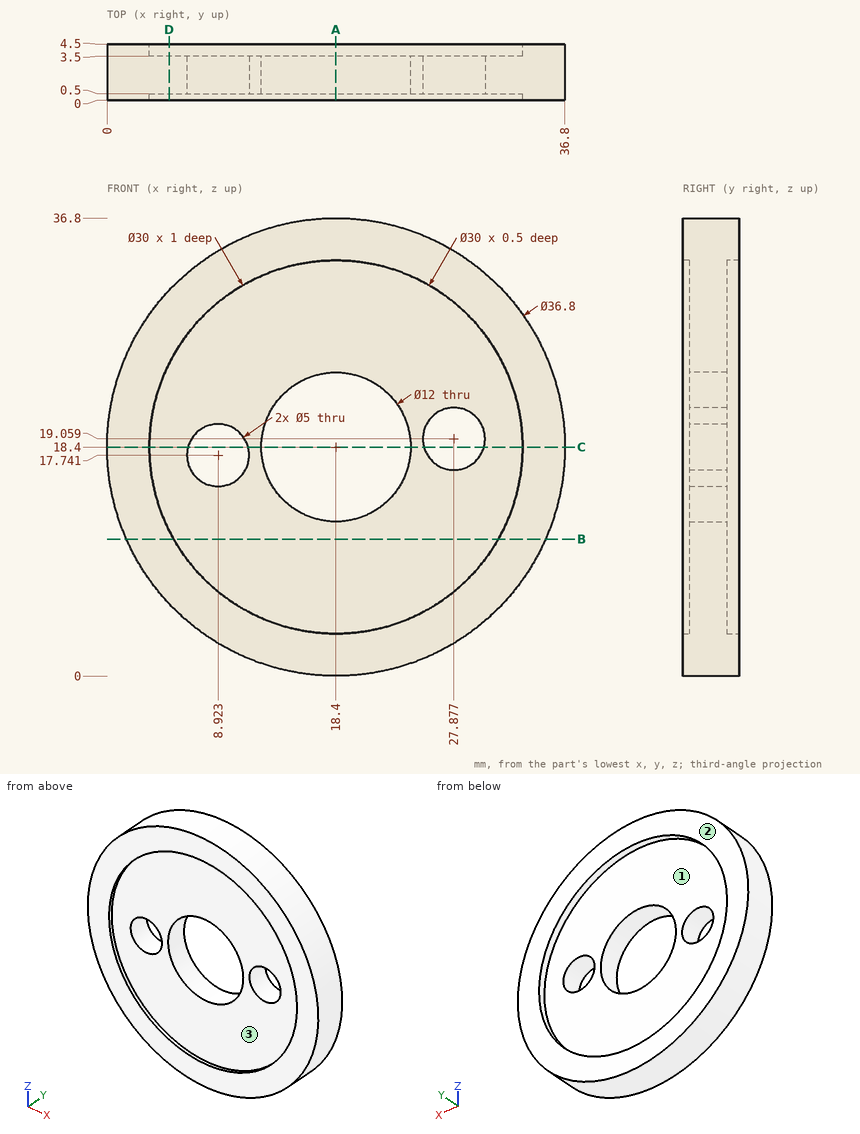
The drawing under review shows one solid part. Ordinate dimensions are in mm from its lowest x, y, z. A direction names the side the tool comes from. Round coordinates to 2 decimals unless told otherwise and drop trailing zeros. Loops run counter-clockwise (first coordinate to the right, second up) from the corner with the lowest first, then second, coordinate; pieces in that order, holes last. Notation, with made-up numbers: (82, -19.75) - (92, -19.75) arc R35 cw to (92, 12.25) - close; hole circle Ø3 at (12, 84). An arc over 180 degrees is marked (long way). One line per question, with ' | ' between items.
1. Clearance check with flat-ended pins moving along their axes: P1, Ø2, axis at y = 1.5, z = 27, coming from the -X side; P2, Ø2, axis at x = 14, y = 4, coming from the -Z side; P3, Ø3, axis at x = 12.5, z = 11, coming from the +Y side. State where each tip first meets the part, or that it passes through.
Results are:
P1: stops at x = 1.64 | P2: stops at z = 0.32 | P3: stops at y = 3.5
2. For the marked faces 1, 2 and 3, list the 3-axis set-ups (+Z, -Z, +X, -X, +Y, -Y) from which the entire face can be reached by the end or side of a thin tool; tool diameter is ignored.
Results are:
face 1: +Y | face 2: +Z, -Z, +X, -X, +Y | face 3: -Y
3. We need section C-C, the plane z = 18.4. State the section outline as (x, y) points (1 decimal).
Results are:
outline: (0, 0) - (3.4, 0) - (3.4, 0.5) - (6.5, 0.5) - (6.5, 3.5) - (3.4, 3.5) - (3.4, 4.5) - (0, 4.5) - close; (11.3, 0.5) - (12.4, 0.5) - (12.4, 3.5) - (11.3, 3.5) - close; (24.4, 0.5) - (25.5, 0.5) - (25.5, 3.5) - (24.4, 3.5) - close; (30.3, 0.5) - (33.4, 0.5) - (33.4, 0) - (36.8, 0) - (36.8, 4.5) - (33.4, 4.5) - (33.4, 3.5) - (30.3, 3.5) - close
4. For L1, parallel to X at y = 3.8, z = 18.4; L2, parallel to Z at x = 19, y = 4.25; L3, parallel to X at y = 2.6, z = 22.5, list the stretches that pass through material, from the lowest coordinate up. Write a range as [from, to].
Results are:
L1: x = [0, 3.4], [33.4, 36.8] | L2: z = [0.01, 3.41], [33.39, 36.79] | L3: x = [0.46, 14.02], [22.78, 36.34]
5. We need section D-D, the plane x = 5. State the section outline as (y, z) points.
Results are:
outline: (0, 5.79) - (4.5, 5.79) - (4.5, 11.66) - (3.5, 11.66) - (3.5, 25.14) - (4.5, 25.14) - (4.5, 31.01) - (0, 31.01) - (0, 25.14) - (0.5, 25.14) - (0.5, 11.66) - (0, 11.66) - close
6. We need section A-A, the plane x = 18.4. State the section outline as (y, z) points.
Results are:
outline: (0, 0) - (4.5, 0) - (4.5, 3.4) - (3.5, 3.4) - (3.5, 12.4) - (0.5, 12.4) - (0.5, 3.4) - (0, 3.4) - close; (0, 33.4) - (0.5, 33.4) - (0.5, 24.4) - (3.5, 24.4) - (3.5, 33.4) - (4.5, 33.4) - (4.5, 36.8) - (0, 36.8) - close
7. We need section B-B, the plane z = 11. State the section outline as (x, y) points.
Results are:
outline: (1.55, 0) - (5.35, 0) - (5.35, 0.5) - (31.45, 0.5) - (31.45, 0) - (35.25, 0) - (35.25, 4.5) - (31.45, 4.5) - (31.45, 3.5) - (5.35, 3.5) - (5.35, 4.5) - (1.55, 4.5) - close
